Work out the finished part from the listing and answer in its coordinate system (mm). Face numbers are marked on the shaded views. A direction names the side the tool comes from. Round coordinates to 2 decimals unless told otherwise and drop trailing zeros. Write each loop counter-clockwise with the first axis right and the second up, starting at its lowest first coordinate (ties: lowest second). Pieces come first, ordered by that corner, then holes. Notation, with made-up numbers: M 31,31.5 L 41,31.5 A12 ccw 41,37.5 Z; hole C -24,-27.75 d6. An arc over 180 degrees is marked long. Answer in a Markdown table with one row per item.
```python
from build123d import *

# Parameters (mm, degrees)
SKETCH_W          = 16
SKETCH_H          = 30
SKETCH_R          = 2.75
PAD_DEPTH         = 7
POCKET_DEPTH      = 4
POCKET_DEPTH_BACK = -4
CHAMFER_SIZE      = 2
SKETCH002_R       = 5
POCKET001_DEPTH   = 4


with BuildPart() as part:
    # Sketch → Pad (new body)
    with BuildSketch(Plane.XY):
        Rectangle(SKETCH_W, SKETCH_H)
        with Locations((0, 7.5)):
            Circle(SKETCH_R, mode=Mode.SUBTRACT)
        with Locations((0, -7.5)):
            Circle(SKETCH_R, mode=Mode.SUBTRACT)
    extrude(amount=PAD_DEPTH)

    # Sketch001 → Pocket (cut, two sides)
    with BuildSketch(Plane.XZ) as pocket_sk:
        with BuildLine():
            ThreePointArc((-7, 0.5), (-7.5, 1), (-8, 0.5))
            Line((-8, 0.5), (-8, -1.5))
            Line((-8, -1.5), (0, -1.5))
            Line((8, -1.5), (0, -1.5))
            Line((8, 0.499993), (8, -1.5))
            ThreePointArc((7, 0.5), (7.499996, 0), (8, 0.499993))
            ThreePointArc((7, 0.5), (6.5, 1), (6, 0.5))
            ThreePointArc((5, 0.5), (5.5, 0), (6, 0.5))
            ThreePointArc((5, 0.5), (4.5, 1), (4, 0.5))
            ThreePointArc((3, 0.5), (3.5, 0), (4, 0.5))
            ThreePointArc((3, 0.5), (2.5, 1), (2, 0.5))
            ThreePointArc((1, 0.5), (1.5, 0), (2, 0.5))
            ThreePointArc((1, 0.5), (0.5, 1), (0, 0.5))
            ThreePointArc((-1, 0.5), (-0.5, 0), (0, 0.5))
            ThreePointArc((-1, 0.5), (-1.5, 1), (-2, 0.5))
            ThreePointArc((-3, 0.5), (-2.5, 0), (-2, 0.5))
            ThreePointArc((-3, 0.5), (-3.5, 1), (-4, 0.5))
            ThreePointArc((-5, 0.5), (-4.5, 0), (-4, 0.5))
            ThreePointArc((-5, 0.5), (-5.5, 1), (-6, 0.5))
            ThreePointArc((-7, 0.5), (-6.5, 0), (-6, 0.5))
        make_face()
    extrude(amount=-POCKET_DEPTH, mode=Mode.SUBTRACT)
    extrude(pocket_sk.sketch, amount=-POCKET_DEPTH_BACK, mode=Mode.SUBTRACT)

    # Chamfer
    chamfer_edges = [part.edges().sort_by_distance(p)[0] for p in [
        (8, 15, 3.5),
        (-8, 15, 3.5),
        (-8, -15, 3.5),
        (-8, 0, 7),
        (0, 15, 7),
        (8, -15, 3.5),
        (0, -15, 7),
        (8, 0, 7),
    ]]
    chamfer(chamfer_edges, length=CHAMFER_SIZE)

    # Sketch002 (on DatumPlane) → Pocket001 (cut)
    with BuildSketch(Plane.XY.offset(7)):
        with Locations((0, 7.5)):
            Circle(SKETCH002_R)
        with Locations((0, -7.5)):
            Circle(SKETCH002_R)
    extrude(amount=-POCKET001_DEPTH, mode=Mode.SUBTRACT)


solid = part.part
```
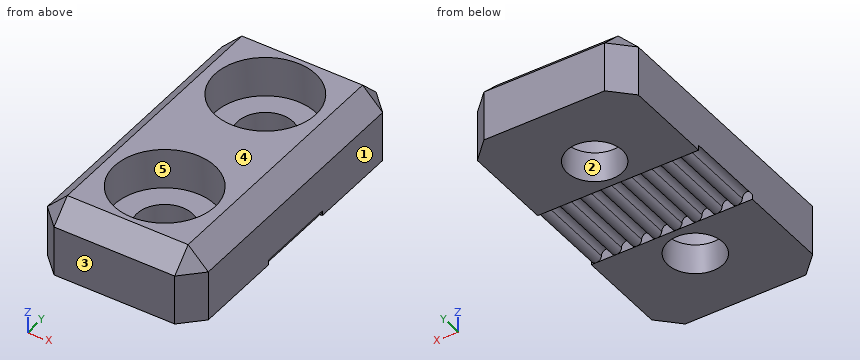
1. Determine the mould class of the marked faces 1, 2 and 3 for opening direction Y: released by +Y, released by -Y, zero draft, split by the parting line, or undercut.
Calculated:
| item | result |
|---|---|
| face 1 | zero draft |
| face 2 | undercut |
| face 3 | released by -Y |
2. The part is cut by section D-D (y = 0.25). Determine the outline of the cut face in (x, z).
Calculated:
| item | result |
|---|---|
| outline | M -8,0.5 A0.5 cw -7,0.5 A0.5 ccw -6,0.5 A0.5 cw -5,0.5 A0.5 ccw -4,0.5 A0.5 cw -3,0.5 A0.5 ccw -2,0.5 A0.5 cw -1,0.5 A0.5 ccw 0,0.5 A0.5 cw 1,0.5 A0.5 ccw 2,0.5 A0.5 cw 3,0.5 A0.5 ccw 4,0.5 A0.5 cw 5,0.5 A0.5 ccw 6,0.5 A0.5 cw 7,0.5 A0.5 ccw 8,0.5 L 8,5 L 6,7 L -6,7 L -8,5 Z |
3. The part is cut by section A-A (y = -7.5). Determine the outline of the cut face in (x, z), plus the area to 3 significant figures.
Calculated:
| item | result |
|---|---|
| outline | M -8,0 L -2.75,0 L -2.75,3 L -5,3 L -5,7 L -6,7 L -8,5 Z; M 2.75,0 L 8,0 L 8,5 L 6,7 L 5,7 L 5,3 L 2.75,3 Z |
| area | 51.5 mm² |
4. The part is cut by section C-C (z = 1.5). Determine the outline of the cut face in (x, y).
Calculated:
| item | result |
|---|---|
| outline | M -8,-13 L -6,-15 L 6,-15 L 8,-13 L 8,13 L 6,15 L -6,15 L -8,13 Z; hole C 0,-7.5 d5.5; hole C 0,7.5 d5.5 |
5. The part is cut by section B-B (x = -5.5). Determine the outline of the cut face in (y, z).
Calculated:
| item | result |
|---|---|
| outline | M -15,0 L -4,0 L -4,1 L 4,1 L 4,0 L 15,0 L 15,5 L 13,7 L -13,7 L -15,5 Z |
6. Consider line 1 along Y through (x, z) = (0, 1.9); line 2 along Y through (x, z) = (0.25, 5.5); line 3 along Z through (x, y) = (-3.25, -6). Determine where each line is inside the solid, lowest interval first. Write a range as from..to.
Calculated:
| item | result |
|---|---|
| line 1 | y = -15..-10.25, -4.75..4.75, 10.25..15 |
| line 2 | y = -14.5..-12.49, -2.51..2.51, 12.49..14.5 |
| line 3 | z = 0..3 |
7. A tool of negligible diameter and unlimited length cuts with its end or side. For the marked faces 4 and 5, from which of +Z, -Z, +X, -X, +Y, -Y can it reach the whole face along a straight path? Write none if from no direction.
Calculated:
| item | result |
|---|---|
| face 4 | +Z, +X, -X, +Y, -Y |
| face 5 | +Z |
8. Given pin 1 (1.1 mm diameter, centred on x = -7.5, z = 0.5, fed in from -Y); pin 2 (0.8 mm diameter, centred on x = 6.5, z = 0.5, fed in from +Y); pin 3 (0.5 mm diameter, centred on x = -7, z = 0.5, fed in from +Y); pin 4 (3.5 mm diameter, centred on x = 0, y = 7.5, fed in from -Z), each flat-ended and moving along its own axis, determine where each tip first touches the part or whether it passes through.
Calculated:
| item | result |
|---|---|
| pin 1 | stops at y = -14.05 |
| pin 2 | stops at y = 14.9 |
| pin 3 | stops at y = 14.25 |
| pin 4 | passes through |
